from build123d import *

# Parameters (mm, degrees)
SKETCH1_R               = 50
BOSS_EXTRUDE1_DEPTH     = 10
SKETCH1_3_R             = 4
CUT_EXTRUDE1_DEPTH      = 10
SKETCH1_4_R             = 20
BOSS_EXTRUDE2_DEPTH     = 62.5
SKETCH4_R               = 15
BOSS_EXTRUDE4_DEPTH     = 50
SKETCH3_R               = 6.5
CUT_EXTRUDE3_DEPTH      = 63.5
CUT_EXTRUDE3_DEPTH_BACK = 11


with BuildPart() as part:
    # Sketch1 → Boss-Extrude1 (new body)
    with BuildSketch(Plane.XY):
        Circle(SKETCH1_R)
    extrude(amount=-BOSS_EXTRUDE1_DEPTH)

    # Sketch1<3> → Cut-Extrude1 (cut)
    with BuildSketch(Plane.XY):
        with Locations((-35, 0)):
            Circle(SKETCH1_3_R)
        with Locations((17.5, 30.310889132)):
            Circle(SKETCH1_3_R)
        with Locations((17.5, -30.310889132)):
            Circle(SKETCH1_3_R)
    extrude(amount=-CUT_EXTRUDE1_DEPTH, mode=Mode.SUBTRACT)

    # Sketch1<4> → Boss-Extrude2 (add)
    with BuildSketch(Plane.XY):
        with Locations((-1.640921825, 0)):
            Circle(SKETCH1_4_R)
        with BuildLine():
            ThreePointArc((-17.320508076, 2.5), (-17.5, 0), (-17.320508076, -2.5))
            Line((-17.320508076, -2.5), (-14.790199458, -2.5))
            ThreePointArc((-14.790199458, -2.5), (15, 0), (-14.790199458, 2.5))
            Line((-14.790199458, 2.5), (-17.320508076, 2.5))
        make_face(mode=Mode.SUBTRACT)
    extrude(amount=BOSS_EXTRUDE2_DEPTH)

    # Sketch4 → Boss-Extrude4 (add)
    with BuildSketch(Plane.XY):
        Circle(SKETCH4_R)
    extrude(amount=BOSS_EXTRUDE4_DEPTH)

    # Sketch3 → Cut-Extrude3 (cut, two sides)
    with BuildSketch(Plane.XY) as cut_extrude3_sk:
        Circle(SKETCH3_R)
    extrude(amount=CUT_EXTRUDE3_DEPTH, mode=Mode.SUBTRACT)
    extrude(cut_extrude3_sk.sketch, amount=-CUT_EXTRUDE3_DEPTH_BACK, mode=Mode.SUBTRACT)


solid = part.part
CAD build for the part. Positions are in the model's coordinates, mm. A direction names the side the tool comes from. Give positions to 0.01 mm unless a question says otherwise; leave off trailing zeros. Order: outer loops, then holes, each group sorted by start corner. A loop starts at its lowest first (then second) coordinate and runs counter-clockwise, first axis right, second up. Notation, with made-up numbers: (14, 76.5) - (56, 76.5) arc R14 cw to (56, 92.5) - close; hole circle Ø11 at (-13.5, -15.75). An arc over 180 degrees is marked (long way). Answer in a Markdown table with one row per item.
1. Saw through at D-D, the plane z = 35. Give the cut face in (x, y).
Data:
| item | result |
|---|---|
| outline | circle Ø40 at (-1.64, 0); hole (-17.32, -2.5) - (-14.79, -2.5) arc R15 cw to (-14.79, 2.5) - (-17.32, 2.5) arc R17.5 ccw to start; hole circle Ø13 at (0, 0) |
2. Saw through at C-C, the plane z = 54.5. Give the cut face in (x, y), plus the area to 3 significant figures.
Data:
| item | result |
|---|---|
| outline | circle Ø40 at (-1.64, 0); hole (-17.32, -2.5) - (-14.79, -2.5) arc R15 ccw (long way) to (-14.79, 2.5) - (-17.32, 2.5) arc R17.5 ccw to start |
| area | 537 mm² |
3. Tool access for faces 1 (the cylindrical face through (17.436, 6.007, 30.812)), 2 (the cylindrical face through (16.979, 34.277, -4.93)): list every direction of +Z, -Z, +X, -X, +Y, -Y with a clear straight run to the whole face (end or side of a thin tool).
Data:
| item | result |
|---|---|
| face 1 | +Z |
| face 2 | +Z, -Z |
4. Probe probe 1 along Y at (x, z) = (17.5, -3.25); probe 2 along Y at (x, z) = (0, -7); probe 3 along Z at (x, y) = (-15, 35.5). List the from-to ranges inside material, lowest first. Write a range as [from, to].
Data:
| item | result |
|---|---|
| probe 1 | y = [-46.84, -34.31], [-26.31, 26.31], [34.31, 46.84] |
| probe 2 | y = [-50, -6.5], [6.5, 50] |
| probe 3 | z = [-10, 0] |
5. Saw through at B-B, the plane y = 0. Give the cut face in (x, z), plus the area to 3 significant figures.
Data:
| item | result |
|---|---|
| outline | (-50, -10) - (-39, -10) - (-39, 0) - (-50, 0) - close; (-31, -10) - (-6.5, -10) - (-6.5, 50) - (-15, 50) - (-15, 0) - (-17.5, 0) - (-17.5, 62.5) - (-21.64, 62.5) - (-21.64, 0) - (-31, 0) - close; (6.5, -10) - (50, -10) - (50, 0) - (18.36, 0) - (18.36, 62.5) - (15, 62.5) - (15, 50) - (6.5, 50) - close |
| area | 2,110 mm² |
6. Pull direction Y, two halves, no side cores. Call faces 3 (the cylindrical face through (47.69, 15.02, -4.93)), 4 (the flat face through (22, 1, 0)), 5 (the cylindrical face through (14.987, -0.624, 56.162)): pulls with the +Y half, pulls with the -Y half, needs draft (parallel to the pull), parting line crosses it, or undercut.
Data:
| item | result |
|---|---|
| face 3 | parting line crosses it |
| face 4 | needs draft |
| face 5 | undercut |
7. Flat gauge pins, fed straight in: pin 1 (8 mm diameter, centred on y = 25, z = 17, fed in from +X); pin 2 (12 mm diameter, centred on x = -7, z = -1.5, fed in from -Y); pin 3 (0.8 mm diameter, centred on x = -16, z = 31.5, fed in from -Y); pin 4 (10.5 mm diameter, centred on x = 17.5, y = 30.31, fed in from +Z). Where does each tip first touch, or does it go through?
Data:
| item | result |
|---|---|
| pin 1 | passes through |
| pin 2 | stops at y = -49.99 |
| pin 3 | stops at y = -14.32 |
| pin 4 | stops at z = 0 |
8. Saw through at A-A, the plane x = -36. Give the cut face in (y, z).
Data:
| item | result |
|---|---|
| outline | (-34.7, -10) - (-3.87, -10) - (-3.87, 0) - (-34.7, 0) - close; (3.87, -10) - (34.7, -10) - (34.7, 0) - (3.87, 0) - close |
